Verification items for the finished model (mm, model axes). A direction names the side the tool comes from. Round coordinates to 2 decimals unless told otherwise and drop trailing zeros. Order: outer loops, then holes, each group sorted by start corner. A loop starts at its lowest first (then second) coordinate and runs counter-clockwise, first axis right, second up. Notation, with made-up numbers: (66, 32) -> (98, 32) arc R28 ccw to (98, 55) -> close; hole circle Ø11 at (49.5, 46.5). An arc over 180 degrees is marked (long way). Put each result on its own line as item: value.
Autodesk Inventor part; units mm, degrees
ref_plane "YZ Plane" through (0, 0, 0) normal (1, 0, 0) x (0, 1, 0)
ref_plane "XZ Plane" through (0, 0, 0) normal (0, 1, 0) x (-1, 0, 0)
ref_plane "XY Plane" through (0, 0, 0) normal (0, 0, 1) x (1, 0, 0)
sketch "Sketch1" plane through (0, 0, 0) normal (1, 0, 0) x (0, 1, 0)
  line L0 (0, 0) -> (9, 0)
  line L1 (9, 0) -> (9, 9)
  line L2 (9, 9) -> (0, 9)
  line L3 (0, 9) -> (0, 0)
  line L4 (9, 8.2) -> (2.5, 8.2)
  line L5 (9, 0.8) -> (2.5, 0.8)
  line L6 (6, 0.8) -> (6, 8.2)
  line L7 (2.5, 0) -> (2.5, 9)
  dimension "d0" = 9
  dimension "d1" = 9
  dimension "d2" = 7.4
  dimension "d3" = 0.8
  dimension "d4" = 2.5
  dimension "d5" = 6
revolve "Revolution1" add sketch "Sketch1" angle 360 about axis through (0, 0, 9) along (0, 0, -1) contours L7 L5 L1 L0 | L7 L4 L6 L5 | L2 L1 L4 L7
properties part number "belt_gear_2"
Item 1: Material ranges on line 1 along X through (y, z) = (0, 6.5); line 2 along Z through (x, y) = (0.75, -6.25); line 3 along Y through (x, z) = (0.5, 8), recorded low to high.
Geometry check:
line 1: -6 to -2.5, 2.5 to 6
line 2: 0 to 0.8, 8.2 to 9
line 3: -5.98 to -2.45, 2.45 to 5.98
Item 2: Depth check by flat-ended pin: pin 1 Ø5.5 at (x, y) = (-2, 3.5) entering from -Z; pin 2 Ø4 at (x, z) = (-5.5, 5) entering from -Y; pin 3 Ø1 at (x, z) = (3, 5.5) entering from +Y; pin 4 Ø1.5 at (y, z) = (-6, 2.5) entering from -X. Enter the tip coordinate at first touch or a pass-through.
Geometry check:
pin 1: z = 0
pin 2: y = -4.87
pin 3: y = 5.45
pin 4: x = -2.9
Item 3: Tool access check on faces 1 (the face through (-2, 2, 0)), 2 (the face through (-6, 2, 0.8)). Record the directions out of +Z, -Z, +X, -X, +Y, -Y that give a thin tool (end or side, any length) a straight path to the whole face; none if there is none.
Geometry check:
face 1: -Z, +X, -X, +Y, -Y
face 2: none
Item 4: Sectioned sample at A-A, the plane x = 0. Record the boundary of the cut face in (y, z), then the cut area to 3 significant figures.
Geometry check:
outline: (-9, 0) -> (-2.5, 0) -> (-2.5, 9) -> (-9, 9) -> (-9, 8.2) -> (-6, 8.2) -> (-6, 0.8) -> (-9, 0.8) -> close; (2.5, 0) -> (9, 0) -> (9, 0.8) -> (6, 0.8) -> (6, 8.2) -> (9, 8.2) -> (9, 9) -> (2.5, 9) -> close
area: 72.6 mm2
Item 5: Release check for a two-part mould opening along Z. For faces 3 (the face through (-6, 2, 8.2)), 4 (the face through (2.44, -0.54, 4.56)), 5 (the face through (-2, 2, 9)) record: pulls with the +Z half, pulls with the -Z half, needs draft (parallel to the pull), parting line crosses it, or undercut.
Geometry check:
face 3: undercut
face 4: needs draft
face 5: pulls with the +Z half
Item 6: Sectioned sample at D-D, the plane y = 7.25. Record the boundary of the cut face in (x, z).
Geometry check:
outline: (-5.33, 0) -> (5.33, 0) -> (5.33, 0.8) -> (-5.33, 0.8) -> close; (-5.33, 8.2) -> (5.33, 8.2) -> (5.33, 9) -> (-5.33, 9) -> close
Item 7: Sectioned sample at C-C, the plane z = 6.75. Record the boundary of the cut face in (x, y).
Geometry check:
outline: circle Ø12 at (0, 0); hole circle Ø5 at (0, 0)
